Can you work these out from the model? Positions are in its coordinate system, mm. A direction names the side the tool comes from. Give positions to 0.01 mm unless a question says otherwise; leave off trailing zeros. Order: outer loops, then holes, each group sorted by start corner. A loop starts at its lowest first (then second) coordinate and runs counter-clockwise, first axis right, second up. Notation, with made-up numbers: (12.25, -29.5) - (45.25, -29.5) arc R20 ccw to (45.25, -13.5) - close; hole circle Ø9 at (-35.75, 12). An arc over 180 degrees is marked (long way). One line per question, with ' | ' between items.
```python
from build123d import *

# Parameters (mm, degrees)
SKETCH1_R           = 2.265
BOSS_EXTRUDE1_DEPTH = 3
SKETCH2_W           = 6.5
SKETCH2_H           = 20
CUT_EXTRUDE1_DEPTH  = 3
BOSS_EXTRUDE2_DEPTH = 3
CUT_EXTRUDE5_DEPTH  = 17
SKETCH9_W           = 65.47
SKETCH9_H           = 1
CUT_EXTRUDE6_DEPTH  = 17
FILLET2_R           = 0.6
FILLET3_R           = 0.1


with BuildPart() as part:
    # Sketch1 → Boss-Extrude1 (new body)
    with BuildSketch(Plane(origin=(0, 0, 0), x_dir=(1, 0, 0), z_dir=(0, 1, 0))):
        with BuildLine():
            Line((4.265, 0), (87.735, 0))
            ThreePointArc((87.735, 0), (95.015810422, 3.015810422), (92, -4.265))
            Line((92, -4.265), (92, -58.735))
            ThreePointArc((92, -58.735), (95.015810422, -66.015810422), (87.735, -63))
            Line((87.735, -63), (4.265, -63))
            ThreePointArc((4.265, -63), (-3.015810422, -66.015810422), (0, -58.735))
            Line((0, -58.735), (0, -4.265))
            ThreePointArc((0, -4.265), (-3.015810422, 3.015810422), (4.265, 0))
        make_face()
        with Locations(Location((0, 0, 0), (0, 0, 270))):
            Circle(SKETCH1_R, mode=Mode.SUBTRACT)
        with Locations(Location((92, 0, 0), (0, 0, 270))):
            Circle(SKETCH1_R, mode=Mode.SUBTRACT)
        with Locations(Location((92, -63, 0), (0, 0, 270))):
            Circle(SKETCH1_R, mode=Mode.SUBTRACT)
        with Locations(Location((0, -63, 0), (0, 0, 270))):
            Circle(SKETCH1_R, mode=Mode.SUBTRACT)
    extrude(amount=BOSS_EXTRUDE1_DEPTH)

    # Sketch2 → Cut-Extrude1 (cut)
    with BuildSketch(Plane(origin=(0, 3, 0), x_dir=(1, 0, 0), z_dir=(0, 1, 0))):
        with Locations((3.25, -31.5)):
            Rectangle(SKETCH2_W, SKETCH2_H)
    extrude(amount=-CUT_EXTRUDE1_DEPTH, mode=Mode.SUBTRACT)

    # Sketch3 → Boss-Extrude2 (add)
    with BuildSketch(Plane(origin=(0, 3, 0), x_dir=(1, 0, 0), z_dir=(0, 1, 0))):
        with BuildLine():
            Line((0, -14.9), (-2.7, -15.5))
            ThreePointArc((-2.7, -15.5), (-2.912132034, -15.587867966), (-3, -15.8))
            Line((-3, -15.8), (-3, -21))
            ThreePointArc((-3, -21), (-2.853553391, -21.353553391), (-2.5, -21.5))
            Line((-2.5, -21.5), (0, -21.5))
            Line((0, -21.5), (0, -14.9))
        make_face()
        with BuildLine():
            Line((0, -41.5), (0, -48.1))
            Line((0, -48.1), (-2.7, -47.5))
            ThreePointArc((-2.7, -47.5), (-2.912132034, -47.412132034), (-3, -47.2))
            Line((-3, -47.2), (-3, -42))
            ThreePointArc((-3, -42), (-2.853553391, -41.646446609), (-2.5, -41.5))
            Line((-2.5, -41.5), (0, -41.5))
        make_face()
    extrude(amount=-BOSS_EXTRUDE2_DEPTH)

    # Sketch8 → Cut-Extrude5 (cut)
    with BuildSketch(Plane(origin=(0, 3, 0), x_dir=(1, 0, 0), z_dir=(0, 1, 0))):
        with BuildLine():
            Line((5, -4.5), (85, -4.5))
            ThreePointArc((85, -4.5), (87.121320344, -5.378679656), (88, -7.5))
            Line((88, -7.5), (88, -58))
            ThreePointArc((88, -58), (87.121320344, -60.121320344), (85, -61))
            Line((85, -61), (5, -61))
            ThreePointArc((5, -61), (2.878679656, -60.121320344), (2, -58))
            Line((2, -58), (2, -7.5))
            ThreePointArc((2, -7.5), (2.878679656, -5.378679656), (5, -4.5))
        make_face()
    extrude(amount=-CUT_EXTRUDE5_DEPTH, mode=Mode.SUBTRACT)

    # Sketch9 → Cut-Extrude6 (cut)
    with BuildSketch(Plane(origin=(0, 3, 0), x_dir=(1, 0, 0), z_dir=(0, 1, 0))):
        with Locations((37, -62.5)):
            Rectangle(SKETCH9_W, SKETCH9_H)
    extrude(amount=-CUT_EXTRUDE6_DEPTH, mode=Mode.SUBTRACT)

    # Fillet2
    fillet2_edges = [part.edges().sort_by_distance(p)[0] for p in [
        (92, 1.5, 4.265),
        (92, 1.5, 58.735),
        (4.265, 1.5, 62),
        (87.735, 1.5, 63),
        (0, 1.5, 58.735),
        (0, 1.5, 4.265),
        (4.265, 1.5, 0),
        (87.735, 1.5, 0),
        (0, 1.5, 14.9),
        (0, 1.5, 48.1),
    ]]
    fillet(fillet2_edges, radius=FILLET2_R)

    # Fillet3
    fillet3_edges = [part.edges().sort_by_distance(p)[0] for p in [
        (69.735, 1.5, 62),
    ]]
    fillet(fillet3_edges, radius=FILLET3_R)


solid = part.part
```
(1) On a 3-axis mill with a long thin cutter (end or side, diameter ignored), from which of +Z, -Z, +X, -X, +Y, -Y can I reach the whole of each face in a straight line? I mean faces 1 (the face through (0, 1, 10)), 2 (the face through (88, 2, 32)). Say none if no direction works.
Answer below:
face 1: -X, +Y, -Y | face 2: +Y, -Y
(2) Will these pins go through, and if not, where does the flat tip stop? pin 1 (0.9 mm diameter, centred on y = 1.5, z = 52, fed in from -X); pin 2 (0.9 mm diameter, centred on y = 1, z = 47.5, fed in from +X); pin 3 (1.5 mm diameter, centred on x = 37.5, y = 1.5, fed in from -Z).
Answer below:
pin 1: x = 0 | pin 2: x = 92 | pin 3: z = 0
(3) If we mould it in two halves opening along Z, with no side actions, what happens to faces 3 (the face through (44, 2, 4.5)), 4 (the face through (37, 2, 62)), 5 (the face through (45, 1, 0))? For each: released by +Z, released by -Z, zero draft, split by the parting line, or undercut.
Answer below:
face 3: undercut | face 4: released by +Z | face 5: released by -Z
(4) Imagine slicing it at A-A (z = 55.5). List the corners of the cut face in (x, y) for me.
Answer below:
outline: (0, 0) - (2, 0) - (2, 3) - (0, 3) - close; (88, 0) - (92, 0) - (92, 3) - (88, 3) - close
(5) If I drill on line 1 (Z direction, x = 82.5, y = 2.4); line 2 (Z direction, x = 49, y = 2.8); line 3 (X direction, y = 1.3, z = 8.5), over which ranges is the centre line in solid material (lowest first)?
Answer below:
line 1: 0 to 4.5, 61 to 63 | line 2: 0 to 4.5, 61 to 62 | line 3: 0 to 2, 88 to 92
(6) Imagine slicing it at B-B (x = 44). List the corners of the cut face in (y, z) for me, and give its area (3 significant figures).
Answer below:
outline: (0, 0) - (3, 0) - (3, 4.5) - (0, 4.5) - close; (0, 61) - (3, 61) - (3, 62) - (0, 62) - close | area: 16.5 mm^2
(7) Imagine slicing it at D-D (z = 34). List the corners of the cut face in (x, y) for me.
Answer below:
outline: (88, 0) - (92, 0) - (92, 3) - (88, 3) - close
(8) Imagine slicing it at C-C (y = 1.95). Count the separate pieces of the cut face and the enclosed holes in it, and give its area (3 significant figures).
Answer below:
separate pieces: 1 | enclosed holes: 4 | area: 984 mm^2
